Read the model definition and answer for the solid it produces. Units are mm, in the model's axes. A direction names the side the tool comes from. Give positions to 0.01 mm unless a question says otherwise; leave off trailing zeros. Order: outer loops, then holes, each group sorted by start corner. A loop starts at its lowest first (then second) coordinate and runs counter-clockwise, first axis right, second up. Notation, with made-up numbers: (-22.5, 34) - (-1.5, 34) arc R21 ccw to (-1.5, 53) - close; hole circle Ø7 at (75.25, 55). An arc over 180 degrees is marked (long way). Use a Markdown table: item, result. Add a question column.
1. Consider L1, parallel to Y at x = 16.5, z = 18.25; L2, parallel to X at y = 19.05, z = 1.7. Determine where each line is inside the solid, lowest interval first.
2. For a pull along Z with two mould halves and no side action, classify faces 1 (the flat face through (21, 0, 13)), 2 (the flat face through (40, 1, 9.416)), 3 (the cylindrical face through (0.955, 1.123, 21.32)) as released by +Z, released by -Z, zero draft, split by the parting line, or undercut.
3. A cutting plane is placed at A-A on y = 15.5. Determine the outline of the cut face in (x, z).
4. Flat-ended cylindrical pins translate along their axes: P1, Ø12, axis at y = 9.5, z = 17, coming from the +X side; P2, Ø8, axis at x = 12.5, y = 18, coming from the +Z side; P3, Ø1.1, axis at y = 3.5, z = 3.5, coming from the -X side; P4, Ø1.8, axis at x = 40.5, y = 1.5, coming from the -Z side. Find the tip coordinate at first contact, or state that the pin passes through.
5. A cutting plane is placed at B-B on x = 28. Determine the outline of the cut face in (y, z) (3 decimals), and give its area (3 significant figures).
6. A cutting plane is placed at C-C on z = 16.75. Determine the outline of the cut face in (x, y) (3 decimals).
7. A cutting plane is placed at D-D on x = 34. Determine the outline of the cut face in (y, z) (3 decimals).
8. Which of the six approach directions +Z, -Z, +X, -X, +Y, -Y give full straight-line access (tool end or side, diameter ignored) to faces 4 (the flat face through (31.432, 3, 3)), 5 (the flat face through (11.112, 3, 3)), 6 (the flat face through (40, 1, 15.766))?
Autodesk Inventor part; units mm, degrees
ref_plane "h1_XY" through (17.4625, 0, 17.526) normal (1, 0, 0) x (0, 0, -1)
ref_plane "h1_YZ" through (17.4625, 0, 17.526) normal (0, 0, -1) x (0, 1, 0)
ref_plane "h1_ZX" through (17.4625, 0, 17.526) normal (0, 1, 0) x (1, 0, 0)
sketch "Sketch_1" plane through (0, 0, 0) normal (1, 0, 0) x (0, 1, 0)
  line L0 (0, 22.225) -> (0, 3.0658)
  arc A0 (0, 3.0658) -> (3.0658, 0) centre (3.0658, 3.0658) ccw
  line L1 (3.0658, 0) -> (31.6408, 0)
  line L2 (31.6408, 0) -> (31.6408, 2.2784)
  line L3 (31.6408, 2.2784) -> (3.0658, 2.2784)
  arc A1 (2.2784, 3.0658) -> (3.0658, 2.2784) centre (3.0658, 3.0658) ccw
  line L4 (2.2784, 3.0658) -> (2.2784, 22.225)
  line L5 (2.2784, 22.225) -> (0, 22.225)
  dimension "d36" = 28.575
  dimension "d37" = 3.0658
  dimension "d38" = 0.7874
  dimension "d40" = 2.2784
  dimension "d43" = 22.225
extrude "Extrusion1" add sketch "Sketch_1" along normal blind 42.545
sketch "Sketch_2" plane through (0, 0, 0) normal (0, 0, 1) x (1, 0, 0)
  line L0 (-3.175, -2.1057) -> (45.72, -2.1057)
  line L1 (45.72, -2.1057) -> (45.72, 33.6906)
  line L2 (45.72, 33.6906) -> (-3.175, 33.6906)
  line L3 (-3.175, 33.6906) -> (-3.175, -2.1057)
  line L4 (-1.905, 0) -> (44.45, 0)
  line L5 (44.45, 0) -> (31.3469, 24.4492)
  arc A0 (31.3469, 24.4492) -> (11.1981, 24.4492) centre (21.2725, 19.05) ccw
  line L6 (11.1981, 24.4492) -> (-1.905, 0)
  line L7 (0, 0) -> (0, 3.0658) construction
  line L8 (0, 3.0658) -> (42.545, 3.0658) construction
  line L9 (42.545, 0) -> (42.545, 3.0658) construction
  line L10 (0, 0) -> (42.545, 0) construction
  line L11 (21.2725, 19.05) -> (21.2725, 0) construction
  line L12 (21.2725, 0) -> (21.2725, -2.1057) construction
  dimension "d23" = 46.355
  dimension "d24" = 11.43
  dimension "d25" = 19.05
  dimension "d26" = 35.7962
  dimension "d27" = 48.895
  dimension "d30" = 2.1057
extrude "Extrusion2" cut sketch "Sketch_2" along normal blind 3.4176
sketch "Sketch3" plane through (42.545, 3.0658, 0) normal (0, 0, -1) x (-1, 0, 0)
  arc A0 (31.3469, 21.3834) -> (11.1981, 21.3834) centre (21.2725, 15.9842) ccw
hole "Drilling 1" at (21.2725, 19.05, 0) direction (0, 0, 1) diameter 16.51 depth 3.4176
sketch "Sketch_8" plane through (0, 0, 0) normal (0, 1, 0) x (-1, 0, 0)
  line L0 (3.4925, 15.7658) -> (-4.7625, 15.7658)
  arc A0 (-4.7625, 15.7658) -> (-4.7625, 9.4158) centre (-4.7625, 12.5908) ccw
  line L1 (-4.7625, 9.4158) -> (3.4925, 9.4158)
  line L2 (3.4925, 9.4158) -> (3.4925, 15.7658)
  line L3 (0, 3.0658) -> (-42.545, 3.0658)
  dimension "d31" = 3.4925
  dimension "d32" = 8.255
  dimension "d33" = 3.175
  dimension "d34" = 6.35
  dimension "d35" = 6.35
extrude "Extrusion5" cut sketch "Sketch_8" along normal blind 3.4176
sketch "Sketch_10" plane through (11.1125, 0, 0) normal (1, 0, 0) x (0, 0, -1)
  arc A0 (-4.5568, 1.8456) -> (-1.8456, 4.5568) centre (-3.0658, 3.0658) ccw
  line L0 (-1.8456, 4.5568) -> (-2.2784, 4.5568)
  line L1 (-2.2784, 4.5568) -> (-4.5568, 2.2784)
  line L2 (-4.5568, 2.2784) -> (-4.5568, 1.8456)
extrude "Extrusion7" add sketch "Sketch_10" along normal blind 2.2784
ref_plane "h1_XY" through (17.4625, 0, 17.526) normal (1, 0, 0) x (0, 0, -1)
ref_plane "h1_YZ" through (17.4625, 0, 17.526) normal (0, 0, -1) x (0, 1, 0)
ref_plane "h1_ZX" through (17.4625, 0, 17.526) normal (0, 1, 0) x (1, 0, 0)
ref_plane "d1_XY" through (17.4625, 8.6728, 0) normal (1, 0, 0) x (0, 0, -1)
ref_plane "d1_YZ" through (17.4625, 8.6728, 0) normal (0, 0, -1) x (0, 1, 0)
ref_plane "d1_ZX" through (17.4625, 8.6728, 0) normal (0, 1, 0) x (1, 0, 0)
ref_plane "h2_XY" through (17.4625, 2.2784, 17.526) normal (1, 0, 0) x (0, 0, -1)
ref_plane "h2_YZ" through (17.4625, 2.2784, 17.526) normal (0, 0, -1) x (0, 1, 0)
ref_plane "h2_ZX" through (17.4625, 2.2784, 17.526) normal (0, 1, 0) x (1, 0, 0)
ref_plane "d2_XY" through (17.4625, 19.8615, 0) normal (1, 0, 0) x (0, 0, -1)
ref_plane "d2_YZ" through (17.4625, 19.8615, 0) normal (0, 0, -1) x (0, 1, 0)
ref_plane "d2_ZX" through (17.4625, 19.8615, 0) normal (0, 1, 0) x (1, 0, 0)
ref_plane "h3_XY" through (17.4625, 14.2672, 2.2784) normal (1, 0, 0) x (0, 0, -1)
ref_plane "h3_YZ" through (17.4625, 14.2672, 2.2784) normal (0, 0, -1) x (0, 1, 0)
ref_plane "h3_ZX" through (17.4625, 14.2672, 2.2784) normal (0, 1, 0) x (1, 0, 0)
ref_plane "h4_XY" through (17.4625, 21.0566, 2.2784) normal (1, 0, 0) x (0, 0, -1)
ref_plane "h4_YZ" through (17.4625, 21.0566, 2.2784) normal (0, 0, -1) x (0, 1, 0)
ref_plane "h4_ZX" through (17.4625, 21.0566, 2.2784) normal (0, 1, 0) x (1, 0, 0)
ref_plane "h5_XY" through (34.925, 3.175, 0) normal (1, 0, 0) x (0, 0, -1)
ref_plane "h5_YZ" through (34.925, 3.175, 0) normal (0, 0, -1) x (0, 1, 0)
ref_plane "h5_ZX" through (34.925, 3.175, 0) normal (0, 1, 0) x (1, 0, 0)
ref_plane "h6_XY" through (34.925, 0, 0) normal (1, 0, 0) x (0, 0, -1)
ref_plane "h6_YZ" through (34.925, 0, 0) normal (0, 0, -1) x (0, 1, 0)
ref_plane "h6_ZX" through (34.925, 0, 0) normal (0, 1, 0) x (1, 0, 0)
ref_plane "l1_XY" through (0, 0, 0) normal (0, 1, 0) x (1, 0, 0)
ref_plane "l1_YZ" through (0, 0, 0) normal (1, 0, 0) x (0, 0, -1)
ref_plane "l1_ZX" through (0, 0, 0) normal (0, 0, -1) x (0, 1, 0)
ref_plane "l2_XY" through (34.925, 0, 0) normal (0, 1, 0) x (1, 0, 0)
ref_plane "l2_YZ" through (34.925, 0, 0) normal (1, 0, 0) x (0, 0, -1)
ref_plane "l2_ZX" through (34.925, 0, 0) normal (0, 0, -1) x (0, 1, 0)
ref_plane "l3_XY" through (0, 0, 17.526) normal (0, 1, 0) x (1, 0, 0)
ref_plane "l3_YZ" through (0, 0, 17.526) normal (1, 0, 0) x (0, 0, -1)
ref_plane "l3_ZX" through (0, 0, 17.526) normal (0, 0, -1) x (0, 1, 0)
ref_plane "l4_XY" through (0, 0, 9.652) normal (0, 1, 0) x (1, 0, 0)
ref_plane "l4_YZ" through (0, 0, 9.652) normal (1, 0, 0) x (0, 0, -1)
ref_plane "l4_ZX" through (0, 0, 9.652) normal (0, 0, -1) x (0, 1, 0)
ref_plane "l5_XY" through (4.7625, 0, 9.652) normal (0, 1, 0) x (1, 0, 0)
ref_plane "l5_YZ" through (4.7625, 0, 9.652) normal (1, 0, 0) x (0, 0, -1)
ref_plane "l5_ZX" through (4.7625, 0, 9.652) normal (0, 0, -1) x (0, 1, 0)
ref_plane "l6_XY" through (30.1625, 0, 9.652) normal (0, 1, 0) x (1, 0, 0)
ref_plane "l6_YZ" through (30.1625, 0, 9.652) normal (1, 0, 0) x (0, 0, -1)
ref_plane "l6_ZX" through (30.1625, 0, 9.652) normal (0, 0, -1) x (0, 1, 0)
ref_plane "l7_XY" through (30.1625, 0, 12.0904) normal (0, 1, 0) x (1, 0, 0)
ref_plane "l7_YZ" through (30.1625, 0, 12.0904) normal (1, 0, 0) x (0, 0, -1)
ref_plane "l7_ZX" through (30.1625, 0, 12.0904) normal (0, 0, -1) x (0, 1, 0)
ref_plane "l8_XY" through (30.1625, 0, 7.2136) normal (0, 1, 0) x (1, 0, 0)
ref_plane "l8_YZ" through (30.1625, 0, 7.2136) normal (1, 0, 0) x (0, 0, -1)
ref_plane "l8_ZX" through (30.1625, 0, 7.2136) normal (0, 0, -1) x (0, 1, 0)
ref_plane "mounting_bracket_XY" through (17.4625, 14.2672, 2.2784) normal (0, 0, 1) x (1, 0, 0)
ref_plane "mounting_bracket_YZ" through (17.4625, 14.2672, 2.2784) normal (1, 0, 0) x (0, 1, 0)
ref_plane "mounting_bracket_ZX" through (17.4625, 14.2672, 2.2784) normal (0, 1, 0) x (0, 0, 1)
ref_plane "mounting_bracket_1_XY" through (17.4625, 14.2672, 0) normal (0, 0, 1) x (1, 0, 0)
ref_plane "mounting_bracket_1_YZ" through (17.4625, 14.2672, 0) normal (1, 0, 0) x (0, 1, 0)
ref_plane "mounting_bracket_1_ZX" through (17.4625, 14.2672, 0) normal (0, 1, 0) x (0, 0, 1)
fillet "Fillet1" radius 3.175 1 edges at (0, 1.1392, 22.225)
ref_plane "Work Plane56" through (21.2725, 0, 0) normal (1, 0, 0) x (0, 0, -1)
mirror "Mirror2" about plane through (21.2725, 0, 0) normal (1, 0, 0) of "Extrusion5", "Fillet1", "Extrusion7"
equation "\"d33\" = 0.5 * d34"
properties part number "Rebuild Shooter NCDME075-0600 Cylinder Mounting Bracket" material "Steel"
Output values:
| question | item | result |
|---|---|---|
| 1 | L1 | 0 to 2.28 |
| 1 | L2 | 8.3 to 13.02, 29.53 to 34.24 |
| 2 | face 1 | zero draft |
| 2 | face 2 | undercut |
| 2 | face 3 | released by +Z |
| 3 | outline | (6.4, 0) - (13.82, 0) - (13.82, 2.28) - (6.4, 2.28) - close; (28.73, 0) - (36.14, 0) - (36.14, 2.28) - (28.73, 2.28) - close |
| 4 | P1 | through |
| 4 | P2 | z = 2.28 |
| 4 | P3 | x = 11.11 |
| 4 | P4 | z = 0.07 |
| 5 | outline | (0, 3.066) arc R3.066 ccw to (3.066, 0) - (14.266, 0) - (14.266, 2.278) - (3.066, 2.278) arc R0.787 cw to (2.278, 3.066) - (2.278, 22.225) - (0, 22.225) - close; (23.834, 0) - (28.29, 0) - (28.29, 2.278) - (23.834, 2.278) - close |
| 5 | area | 86.2 mm² |
| 6 | outline | (0, 0) - (42.545, 0) - (42.545, 2.278) - (0, 2.278) - close |
| 7 | outline | (0, 3.066) arc R3.066 ccw to (3.066, 0) - (19.499, 0) - (19.499, 2.278) - (3.066, 2.278) arc R0.787 cw to (2.278, 3.066) - (2.278, 22.225) - (0, 22.225) - close |
| 8 | face 4 | +Z, +X, +Y |
| 8 | face 5 | +Z, -X, +Y |
| 8 | face 6 | +X, +Y, -Y |
